```python
from build123d import *

# Parameters (mm, degrees)
SKETCH2_W           = 10
SKETCH2_H           = 10
SKETCH2_R           = 1.5
SKETCH2_W_2         = 12.62
SKETCH2_H_2         = 13.97
SKETCH2_W_3         = 2
SKETCH2_H_3         = 8
BOSS_EXTRUDE1_DEPTH = 3
FILLET2_R           = 1
FILLET3_R           = 1


with BuildPart() as part:
    # Sketch2 → Boss-Extrude1 (new body)
    # profile 1 of 3: a face of its own
    with BuildSketch(Plane(origin=(0, 0, 0), x_dir=(1, 0, 0), z_dir=(0, 1, 0))):
        with Locations((7.62, -5)):
            Rectangle(SKETCH2_W, SKETCH2_H)
        with Locations(Location((7.62, -5, 0), (0, 0, 270))):
            Circle(SKETCH2_R, mode=Mode.SUBTRACT)
    # profile 2 of 3: a face of its own
    with BuildSketch(Plane(origin=(0, 0, 0), x_dir=(1, 0, 0), z_dir=(0, 1, 0))):
        with Locations((6.31, 6.985)):
            Rectangle(SKETCH2_W_2, SKETCH2_H_2)
        with Locations(Location((7.62, 6.985, 0), (0, 0, 270))):
            Circle(SKETCH2_R, mode=Mode.SUBTRACT)
        with Locations((2.54, 6.985)):
            Rectangle(SKETCH2_W_3, SKETCH2_H_3, mode=Mode.SUBTRACT)
    # profile 3 of 3: a face of its own
    with BuildSketch(Plane(origin=(0, 0, 0), x_dir=(1, 0, 0), z_dir=(0, 1, 0))):
        with Locations((7.62, 18.97)):
            Rectangle(SKETCH2_W, SKETCH2_H)
        with Locations(Location((7.62, 18.97, 0), (0, 0, 270))):
            Circle(SKETCH2_R, mode=Mode.SUBTRACT)
    extrude(amount=BOSS_EXTRUDE1_DEPTH)

    # Fillet2
    fillet2_edges = [part.edges().sort_by_distance(p)[0] for p in [
        (1.54, 1.5, -2.985),
        (3.54, 1.5, -2.985),
        (3.54, 1.5, -10.985),
        (1.54, 1.5, -10.985),
    ]]
    fillet(fillet2_edges, radius=FILLET2_R - 0.0001)  # a hair under: the kernel refuses the full size

    # Fillet3
    fillet3_edges = [part.edges().sort_by_distance(p)[0] for p in [
        (12.62, 1.5, 10),
        (2.62, 1.5, 10),
        (2.62, 1.5, 0),
        (0, 1.5, 0),
        (0, 1.5, -13.97),
        (2.62, 1.5, -13.97),
        (2.62, 1.5, -23.97),
        (12.62, 1.5, -23.97),
    ]]
    fillet(fillet3_edges, radius=FILLET3_R)


solid = part.part
```
Input: part model. Units: mm. Frame: model coordinates. A direction names the side the tool comes from. Round coordinates to 2 decimals unless told otherwise and drop trailing zeros. Loops run counter-clockwise (first coordinate to the right, second up) from the corner with the lowest first, then second, coordinate; pieces in that order, holes last. Notation, with made-up numbers: M 24.5,-32.5 L 55.5,-32.5 A25 cw 55.5,-1.5 Z; hole C 57.5,-13.75 d6. An arc over 180 degrees is marked long. Answer in a Markdown table with one row per item. Add a question column.
1. Section C-C (y = 2.6). Give the number of separate pieces and of enclosed holes in the cut face, and give its area (3 significant figures).
2. Section A-A (x = 7.62). Output: boundary loops of the cut face in (y, z) (3 decimals).
3. Contact query for flat-ended pins moving along their axis: pin 1 (0.7 mm diameter, centred on x = 1.5, y = 2, fed in from -Z); pin 2 (1.5 mm diameter, centred on y = 2, z = -18.5, fed in from -X); pin 3 (2.5 mm diameter, centred on x = 7.62, z = -6.985, fed in from -Y); pin 4 (0.7 mm diameter, centred on x = 1.5, y = 2, fed in from +Z). Output: stop coordinate, or through.
4. Ray query, probe 1 along X at (y, z) = (0.65, 5); probe 2 along X at (y, z) = (2.6, -9.5); probe 3 along X at (y, z) = (2.05, -6.5). Return the intervals inside material, ascending.
5. Section D-D (x = 3). Output: boundary loops of the cut face in (y, z).
6. Section B-B (z = 5). Output: boundary loops of the cut face in (x, y), and give its area (3 significant figures).
7. Set-up query: faces 5 (the face through (3.255, 1.521, -3.286)), 6 (the face through (12.319, 1.521, 9.715)), 7 (the face through (2.62, 1, 5)). Return all of +Z, -Z, +X, -X, +Y, -Y with unobstructed straight access to the full face (end or side cutting, diameter ignored); none if empty.
8. Mould query, pull axis Z, two halves, no side actions, for faces 1 (the face through (0, 1, -7)), 2 (the face through (8, 1, 10)), 3 (the face through (2.905, 1.521, -23.669)), 4 (the face through (6.29, 1.48, 5.69)). Classes: released by +Z, released by -Z, zero draft, split by the parting line, or undercut.
Values follow:
| question | item | result |
|---|---|---|
| 1 | separate pieces | 1 |
| 1 | enclosed holes | 4 |
| 1 | area | 339 mm^2 |
| 2 | outline | M 0,-23.97 L 3,-23.97 L 3,-20.47 L 0,-20.47 Z; M 0,-17.47 L 3,-17.47 L 3,-8.485 L 0,-8.485 Z; M 0,-5.485 L 3,-5.485 L 3,3.5 L 0,3.5 Z; M 0,6.5 L 3,6.5 L 3,10 L 0,10 Z |
| 3 | pin 1 | z = -14 |
| 3 | pin 2 | x = 2.62 |
| 3 | pin 3 | through |
| 3 | pin 4 | z = 0.03 |
| 4 | probe 1 | 2.62 to 6.12, 9.12 to 12.62 |
| 4 | probe 2 | 0 to 1.54, 3.54 to 12.62 |
| 4 | probe 3 | 0 to 1.54, 3.54 to 6.2, 9.04 to 12.62 |
| 5 | outline | M 0,-23.75 L 3,-23.75 L 3,-10.87 L 0,-10.87 Z; M 0,-3.1 L 3,-3.1 L 3,9.78 L 0,9.78 Z |
| 6 | outline | M 2.62,0 L 6.12,0 L 6.12,3 L 2.62,3 Z; M 9.12,0 L 12.62,0 L 12.62,3 L 9.12,3 Z |
| 6 | area | 21.0 mm^2 |
| 7 | face 5 | +Y, -Y |
| 7 | face 6 | +Z, +X, +Y, -Y |
| 7 | face 7 | +Z, -X, +Y, -Y |
| 8 | face 1 | zero draft |
| 8 | face 2 | released by +Z |
| 8 | face 3 | released by -Z |
| 8 | face 4 | undercut |
